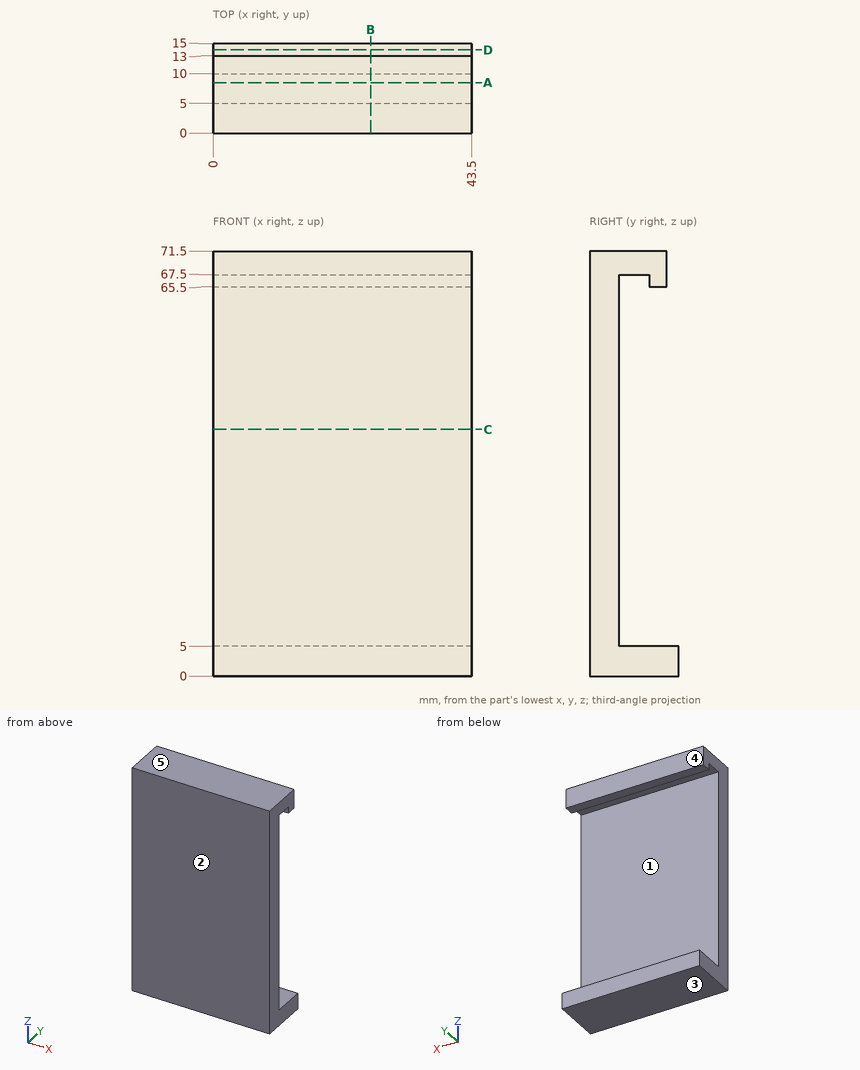
Can you work these out from the drawing? Everything is in mm from the part's minimum corner. A direction names the side the tool comes from. Give positions to 0.01 mm unless a question says otherwise; leave off trailing zeros. Loops run counter-clockwise (first coordinate to the right, second up) from the corner with the lowest first, then second, coordinate; pieces in that order, holes last. Notation, with made-up numbers: (-30, 14) -> (-10, 14) arc R25 ccw to (-10, 41) -> close; hole circle Ø4 at (3.5, 72.5). An arc over 180 degrees is marked (long way). Return JSON: item names as keys, results as strings.
Q1. We'd pull the mould along Z, two halves only. Please class the marked faces 1, 2 and 3: released by +Z, released by -Z, zero draft, split by the parting line, or undercut.
Checks:
{"face 1": "undercut", "face 2": "zero draft", "face 3": "released by -Z"}
Q2. On a 3-axis mill with a long thin cutter (end or side, diameter ignored), from which of +Z, -Z, +X, -X, +Y, -Y can I reach the whole of each face in a straight line? I mean the marked faces 4 and 5. Say none if no direction works.
Checks:
{"face 4": "+Z, +X, -X, +Y", "face 5": "+Z, +X, -X, +Y, -Y"}
Q3. I want a section at C-C, the plane z = 41.5. List the corners of the cut face in (x, y) for me.
Checks:
{"outline": "(0, 0) -> (43.5, 0) -> (43.5, 5) -> (0, 5) -> close"}
Q4. I want a section at A-A, the plane y = 8.5. List the corners of the cut face in (x, z) for me, then the cut area to 4 significant figures.
Checks:
{"outline": "(0, 0) -> (43.5, 0) -> (43.5, 5) -> (0, 5) -> close; (0, 67.5) -> (43.5, 67.5) -> (43.5, 71.5) -> (0, 71.5) -> close", "area": "391.5 mm2"}
Q5. I want a section at B-B, the plane x = 26.5. List the corners of the cut face in (y, z) for me.
Checks:
{"outline": "(0, 0) -> (15, 0) -> (15, 5) -> (5, 5) -> (5, 67.5) -> (10, 67.5) -> (10, 65.5) -> (13, 65.5) -> (13, 71.5) -> (0, 71.5) -> close"}
Q6. I need wall thicknesses on probe 1 along Z at (x, y) = (3, 12); probe 2 along Z at (x, y) = (26.5, 9.25); probe 3 along Y at (x, z) = (11, 26.5). Which ranges of each line are inside material? Lowest first, please.
Checks:
{"probe 1": "z = 0 to 5, 65.5 to 71.5", "probe 2": "z = 0 to 5, 67.5 to 71.5", "probe 3": "y = 0 to 5"}
Q7. For pin 1 Ø1.5 at (x, y) = (25.5, 7.5) entering from -Z; pin 2 Ø6.5 at (x, z) = (31, 67.5) entering from +Y; pin 3 Ø1 at (y, z) = (7, 18) entering from +X; pin 4 Ø12 at (x, z) = (35.5, 14.5) entering from +Y, each with a flat end and sliding along its axis, tell me the tip position at first contact or that it passes through.
Checks:
{"pin 1": "stops at z = 0", "pin 2": "stops at y = 13", "pin 3": "passes through", "pin 4": "stops at y = 5"}
